Could you check a few things on this drawing? It's one solid part, dimensions in mm from its lowest x, y, z. A direction names the side the tool comes from. Coordinates: 2 decimals unless noted, no trailing zeros. Order: outer loops, then holes, each group sorted by start corner. A loop starts at its lowest first (then second) coordinate and runs counter-clockwise, first axis right, second up. Notation, with made-up numbers: (84, -39.75) - (127, -39.75) arc R14 ccw to (127, -26.75) - close; hole circle Ø3 at (4, 9). An arc over 180 degrees is marked (long way). Answer in a Markdown table with one row per item. Add a question column.
Item 1: If I drill on line 1 along Y through (x, z) = (30, 3.5); line 2 along X through (y, z) = (64.5, 1.25), over which ranges is the centre line in solid material (lowest first)? Write a range as from..to.
Item 2: On a 3-axis mill with a long thin cutter (end or side, diameter ignored), from which of +Z, -Z, +X, -X, +Y, -Y can I reach the whole of each face in a straight line? I mean the marked faces 4 and 5. Say none if no direction works.
Item 3: I want a section at A-A (y = 11.5). Please give me the cut outline in (x, z), plus the area to 3 significant figures.
Item 4: Thinking about a two-plate mould opening in Y: for the marked faces 1, 2 and 3, which applies, +Y half, -Y half, draft (parallel to the pull), parting line (faces both ways), or undercut?
Item 5: I want a section at B-B (z = 3.75). Please give me the cut outline in (x, y), plus the area to 3 significant figures.
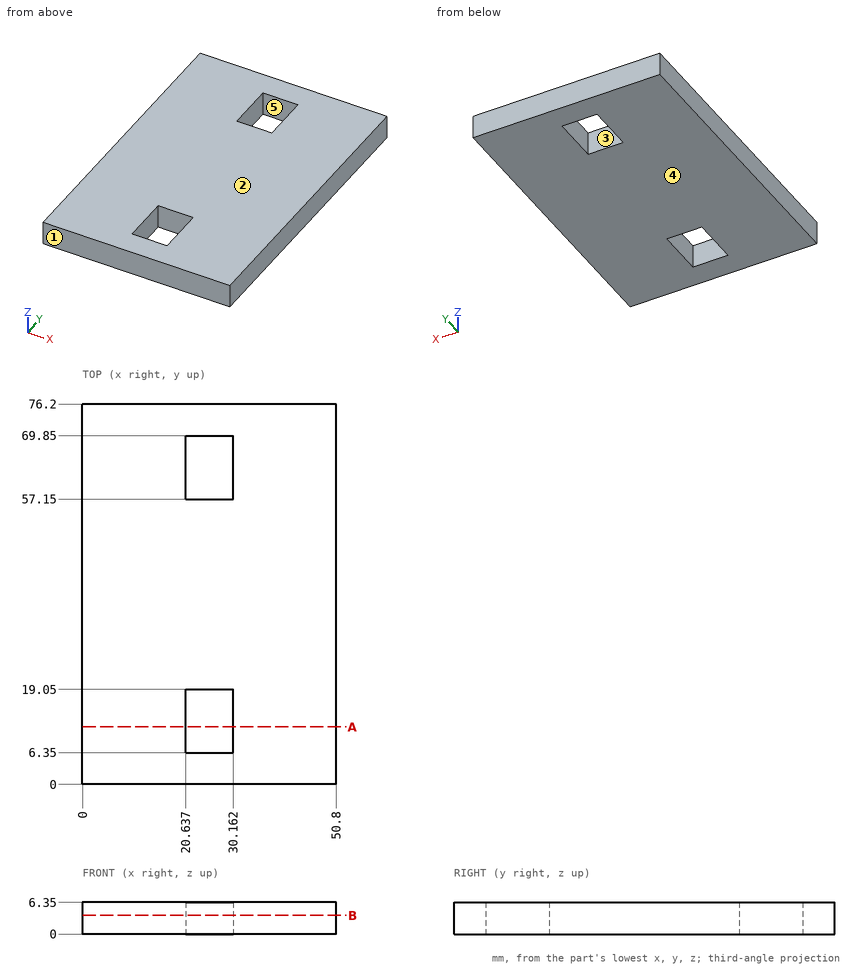
Values follow:
| question | item | result |
|---|---|---|
| 1 | line 1 | y = 0..6.35, 19.05..57.15, 69.85..76.2 |
| 1 | line 2 | x = 0..20.64, 30.16..50.8 |
| 2 | face 4 | -Z, +X, -X, +Y, -Y |
| 2 | face 5 | +Z, -Z |
| 3 | outline | (0, 0) - (20.64, 0) - (20.64, 6.35) - (0, 6.35) - close; (30.16, 0) - (50.8, 0) - (50.8, 6.35) - (30.16, 6.35) - close |
| 3 | area | 262 mm^2 |
| 4 | face 1 | -Y half |
| 4 | face 2 | draft |
| 4 | face 3 | undercut |
| 5 | outline | (0, 0) - (50.8, 0) - (50.8, 76.2) - (0, 76.2) - close; hole (20.64, 6.35) - (30.16, 6.35) - (30.16, 19.05) - (20.64, 19.05) - close; hole (20.64, 57.15) - (30.16, 57.15) - (30.16, 69.85) - (20.64, 69.85) - close |
| 5 | area | 3,630 mm^2 |
